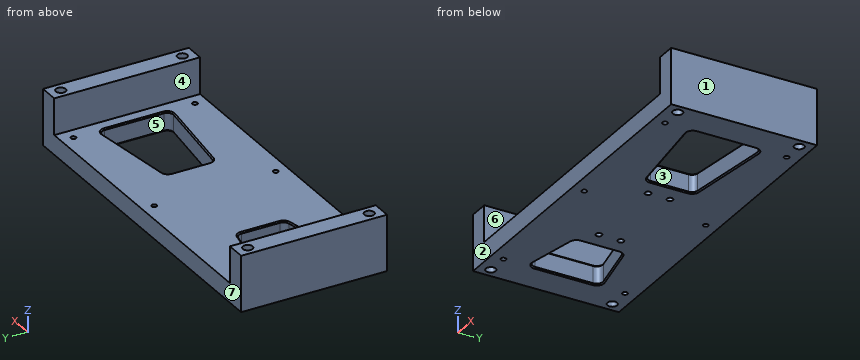
from build123d import *

# Parameters (mm, degrees)
SKETCH1_W                   = 282
SKETCH1_H                   = 16
BOSS_EXTRUDE1_DEPTH         = 120
SKETCH4_W                   = 16
SKETCH4_H                   = 120
BOSS_EXTRUDE2_DEPTH         = 30
SKETCH2_R                   = 4
CUT_EXTRUDE1_DEPTH          = 278.546392518
M5_TAPPED_HOLE1_D           = 4.2
TAP_DRILL_FOR_M6_TAP1_D     = 5
TAP_DRILL_FOR_M6_TAP1_DEPTH = 8
TAP_DRILL_FOR_M6_TAP1_TIP   = 1.502151548
CUT_EXTRUDE2_DEPTH          = 278.546392518
CHAMFER1_SIZE               = 1


with BuildPart() as part:
    # Sketch1 → Boss-Extrude1 (new body)
    with BuildSketch(Plane(origin=(0, 0, 0), x_dir=(1, 0, 0), z_dir=(0, 1, 0))):
        with Locations((105, 38)):
            Rectangle(SKETCH1_W, SKETCH1_H)
    extrude(amount=BOSS_EXTRUDE1_DEPTH)

    # Sketch4 → Boss-Extrude2 (add)
    with BuildSketch(Plane.XY.offset(-30)):
        with Locations((-28, 60)):
            Rectangle(SKETCH4_W, SKETCH4_H)
        with Locations((238, 60)):
            Rectangle(SKETCH4_W, SKETCH4_H)
    extrude(amount=BOSS_EXTRUDE2_DEPTH)

    # Sketch2 → Cut-Extrude1 (cut, through all)
    with BuildSketch(Plane.XY.offset(-46)):
        with Locations(Location((238, 110, 0), (0, 0, 180))):
            Circle(SKETCH2_R)
        with Locations(Location((-28, 110, 0), (0, 0, 180))):
            Circle(SKETCH2_R)
        with Locations(Location((-28, 10, 0), (0, 0, 180))):
            Circle(SKETCH2_R)
        with Locations(Location((238, 10, 0), (0, 0, 180))):
            Circle(SKETCH2_R)
    extrude(amount=CUT_EXTRUDE1_DEPTH, mode=Mode.SUBTRACT)

    # M5 Tapped Hole1 (through all)
    with Locations(Plane.XY.offset(-30)):
        with Locations((-10, 110), (105, 110), (220, 110), (220, 10), (105, 10), (-10, 10)):
            Hole(M5_TAPPED_HOLE1_D / 2)

    # Tap Drill for M6 Tap1
    with Locations(Plane(origin=(0, 0, -46), x_dir=(-1, 0, 0), z_dir=(0, 0, -1))):
        with Locations((-55, 51), (-55, 69), (-125, 69), (-125, 51)):
            Hole(TAP_DRILL_FOR_M6_TAP1_D / 2, depth=TAP_DRILL_FOR_M6_TAP1_DEPTH)
            with Locations((0, 0, -(TAP_DRILL_FOR_M6_TAP1_DEPTH + TAP_DRILL_FOR_M6_TAP1_TIP / 2))):  # 118° drill point
                Cone(0, TAP_DRILL_FOR_M6_TAP1_D / 2, TAP_DRILL_FOR_M6_TAP1_TIP, mode=Mode.SUBTRACT)

    # Sketch11 → Cut-Extrude2 (cut, through all)
    with BuildSketch(Plane(origin=(0, 0, -46), x_dir=(-1, 0, 0), z_dir=(0, 0, -1))):
        with BuildLine():
            Line((-140, 75.586088907), (-140, 44.413911093))
            ThreePointArc((-140, 44.413911093), (-141.251609121, 41.104898277), (-144.379826327, 39.452521709))
            Line((-144.379826327, 39.452521709), (-214.379826327, 30.702521709))
            ThreePointArc((-214.379826327, 30.702521709), (-218.309012816, 31.915520214), (-220, 35.663911093))
            Line((-220, 35.663911093), (-220, 84.336088907))
            ThreePointArc((-220, 84.336088907), (-218.309012816, 88.084479786), (-214.379826327, 89.297478291))
            Line((-214.379826327, 89.297478291), (-144.379826327, 80.547478291))
            ThreePointArc((-144.379826327, 80.547478291), (-141.251609121, 78.895101723), (-140, 75.586088907))
        make_face()
        with BuildLine():
            Line((10, 83.900980486), (10, 36.099019514))
            ThreePointArc((10, 36.099019514), (8.169944528, 32.232308807), (4.019419324, 31.196116135))
            Line((4.019419324, 31.196116135), (-35.980580676, 39.196116135))
            ThreePointArc((-35.980580676, 39.196116135), (-38.866710707, 40.929074986), (-40, 44.099019514))
            Line((-40, 44.099019514), (-40, 75.900980486))
            ThreePointArc((-40, 75.900980486), (-38.866710707, 79.070925014), (-35.980580676, 80.803883865))
            Line((-35.980580676, 80.803883865), (4.019419324, 88.803883865))
            ThreePointArc((4.019419324, 88.803883865), (8.169944528, 87.767691193), (10, 83.900980486))
        make_face()
    extrude(amount=-CUT_EXTRUDE2_DEPTH, mode=Mode.SUBTRACT)

    # Chamfer1
    chamfer1_edges = [part.edges().sort_by_distance(p)[0] for p in [
        (141.251609121, 41.104898277, -30),
        (179.379826327, 35.077521709, -30),
        (218.309012816, 31.915520214, -30),
        (220, 60, -30),
        (218.309012816, 88.084479786, -30),
        (179.379826327, 84.922478291, -30),
        (141.251609121, 78.895101723, -30),
        (140, 60, -30),
        (141.251609121, 41.104898277, -46),
        (140, 60, -46),
        (141.251609121, 78.895101723, -46),
        (179.379826327, 84.922478291, -46),
        (218.309012816, 88.084479786, -46),
        (220, 60, -46),
        (218.309012816, 31.915520214, -46),
        (179.379826327, 35.077521709, -46),
        (-8.169944528, 32.232308807, -30),
        (15.980580676, 35.196116135, -30),
        (38.866710707, 40.929074986, -30),
        (40, 60, -30),
        (38.866710707, 79.070925014, -30),
        (15.980580676, 84.803883865, -30),
        (-8.169944528, 87.767691193, -30),
        (-10, 60, -30),
        (-8.169944528, 32.232308807, -46),
        (-10, 60, -46),
        (-8.169944528, 87.767691193, -46),
        (15.980580676, 84.803883865, -46),
        (38.866710707, 79.070925014, -46),
        (40, 60, -46),
        (38.866710707, 40.929074986, -46),
        (15.980580676, 35.196116135, -46),
    ]]
    chamfer(chamfer1_edges, length=CHAMFER1_SIZE)


solid = part.part
Work out the finished part from the listing and answer in its coordinate system (mm). Face numbers are marked on the shaded views. A direction names the side the tool comes from. Round coordinates to 2 decimals unless told otherwise and drop trailing zeros. Loops run counter-clockwise (first coordinate to the right, second up) from the corner with the lowest first, then second, coordinate; pieces in that order, holes last. Notation, with made-up numbers: (0.5, 69.5) - (32.5, 69.5) arc R14 cw to (32.5, 93.5) - close; hole circle Ø1 at (61.25, 47.5). An arc over 180 degrees is marked (long way). One line per item, written item: value.
Q1. Find section D-D on x = 81. Give the vertices of the cut face in (y, z), and give its area (3 significant figures).
Check values:
outline: (0, -46) - (120, -46) - (120, -30) - (0, -30) - close
area: 1,920 mm2
Q2. Find section A-A on z = -3.5. Give the vertices of the cut face in (x, y), and give its area (3 significant figures).
Check values:
outline: (-36, 0) - (-20, 0) - (-20, 120) - (-36, 120) - close; (230, 0) - (246, 0) - (246, 120) - (230, 120) - close; hole circle Ø8 at (-28, 10); hole circle Ø8 at (-28, 110); hole circle Ø8 at (238, 10); hole circle Ø8 at (238, 110)
area: 3,640 mm2
Q3. Find section C-C on y = 101.5. Give the vertices of the cut face in (x, z), and give its area (3 significant figures).
Check values:
outline: (-36, -46) - (246, -46) - (246, 0) - (230, 0) - (230, -30) - (-20, -30) - (-20, 0) - (-36, 0) - close
area: 5,470 mm2
Q4. Straight lines are drawn through the part: probe 1 along Y at (x, z) = (238, -10); probe 2 along X at (y, z) = (10, -11); probe 3 along X at (y, z) = (51, -41). For each, find the intervals that lie inside material, in ascending order.
Check values:
probe 1: 0 to 6, 14 to 106, 114 to 120
probe 2: -36 to -32, -24 to -20, 230 to 234, 242 to 246
probe 3: -36 to -10, 40 to 52.5, 57.5 to 122.5, 127.5 to 140, 220 to 246
Q5. The mould has two halves that part along X. Classify the marked faces 1, 2, 3 and 4: +X half, -X half, draft (parallel to the pull), parting line (faces both ways), or undercut.
Check values:
face 1: +X half
face 2: draft
face 3: undercut
face 4: undercut
Q6. Find section B-B on x = 2. Give the vertices of the cut face in (y, z).
Check values:
outline: (0, -46) - (31.38, -46) - (32.4, -45) - (32.4, -31) - (31.38, -30) - (0, -30) - close; (87.6, -45) - (88.62, -46) - (120, -46) - (120, -30) - (88.62, -30) - (87.6, -31) - close
Q7. Each of these flat-tipped pins is pushed along its axis until it touches: pin 1 Ø4 at (x, y) = (125, 51) entering from +Z; pin 2 Ø1.5 at (x, z) = (95.5, -29) entering from +Y. Where does it stop, or does it pass through?
Check values:
pin 1: z = -30
pin 2: through
Q8. For the marked faces 5, 6 and 7, determine the directions among +Z, -Z, +X, -X, +Y, -Y from which every point of the face is accessible in a straight line to the end or side of a thin tool.
Check values:
face 5: +Z, -Z
face 6: +Z, +Y, -Y
face 7: +Z, -Z, +X, -X, +Y
